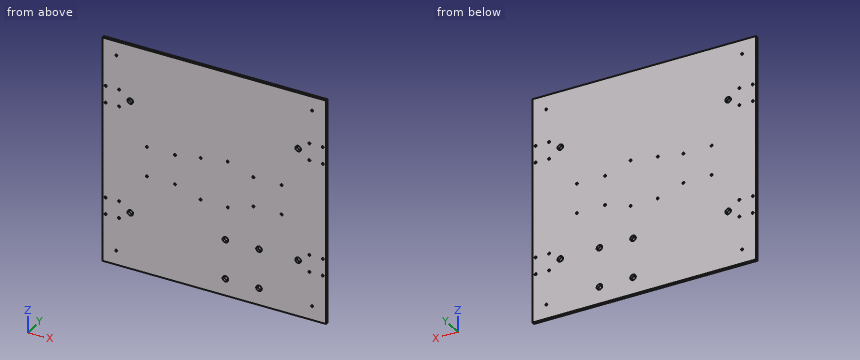
Autodesk Inventor part; units mm, degrees
ref_plane "YZ Plane" through (0, 0, 0) normal (1, 0, 0) x (0, 1, 0)
ref_plane "XZ Plane" through (0, 0, 0) normal (0, 1, 0) x (-1, 0, 0)
ref_plane "XY Plane" through (0, 0, 0) normal (0, 0, 1) x (1, 0, 0)
sketch "草图1" plane through (0, 0, 0) normal (0, 1, 0) x (-1, 0, 0)
  line L0 (200, 200) -> (-200, 200)
  line L1 (-200, 200) -> (-200, -200)
  line L2 (-200, -200) -> (200, -200)
  line L3 (200, -200) -> (200, 200)
  point P0 (0, 0)
  dimension "d0" = 400
  dimension "d1" = 400
extrude "拉伸1" add sketch "草图1" along normal blind 5
sketch "草图2" plane through (0, 5, 0) normal (0, 1, 0) x (1, 0, 0)
  circle A0 centre (175, 175) radius 1.8
  point P0 (0, 0)
  dimension "d4" = 3.6
extrude "拉伸2" cut sketch "草图2" against normal through all
sketch "草图3" plane through (0, 0, 0) normal (0, -1, 0) x (1, 0, 0)
  circle A0 centre (175, 175) radius 1.8
  point P0 (0, 0)
  dimension "d7" = 3.6
extrude "拉伸3" cut sketch "草图3" against normal through all
sketch "草图4" plane through (0, 0, 0) normal (0, -1, 0) x (1, 0, 0)
  circle A0 centre (-175, -175) radius 1.8
  point P0 (0, 0)
  dimension "d10" = 3.6
extrude "拉伸4" cut sketch "草图4" against normal through all
sketch "草图5" plane through (0, 0, 0) normal (0, -1, 0) x (1, 0, 0)
  circle A0 centre (-175, 175) radius 1.8
  point P0 (0, 0)
  dimension "d13" = 3.6
extrude "拉伸5" cut sketch "草图5" against normal through all
sketch "草图6" plane through (0, 0, 0) normal (0, -1, 0) x (1, 0, 0)
  circle A0 centre (-194, -85) radius 1.8
  point P0 (0, 0)
  dimension "d16" = 3.6
extrude "拉伸6" cut sketch "草图6" against normal through all
sketch "草图7" plane through (0, 0, 0) normal (0, -1, 0) x (1, 0, 0)
  circle A0 centre (-170, -85) radius 1.8
  point P0 (0, 0)
  dimension "d19" = 3.6
extrude "拉伸7" cut sketch "草图7" against normal through all
sketch "草图8" plane through (0, 0, 0) normal (0, -1, 0) x (1, 0, 0)
  circle A0 centre (-194, -115) radius 1.8
  point P0 (0, 0)
  dimension "d22" = 3.6
extrude "拉伸8" cut sketch "草图8" against normal through all
sketch "草图9" plane through (0, 0, 0) normal (0, -1, 0) x (1, 0, 0)
  circle A0 centre (-170, -115) radius 1.8
  point P0 (0, 0)
  dimension "d25" = 3.6
extrude "拉伸9" cut sketch "草图9" against normal through all
sketch "草图10" plane through (0, 0, 0) normal (0, -1, 0) x (1, 0, 0)
  circle A0 centre (194, 85) radius 1.8
  point P0 (0, 0)
  dimension "d28" = 3.6
extrude "拉伸10" cut sketch "草图10" against normal through all
sketch "草图11" plane through (0, 0, 0) normal (0, -1, 0) x (1, 0, 0)
  circle A0 centre (194, 115) radius 1.8
  point P0 (0, 0)
  dimension "d31" = 3.6
extrude "拉伸11" cut sketch "草图11" against normal through all
sketch "草图12" plane through (0, 0, 0) normal (0, -1, 0) x (1, 0, 0)
  circle A0 centre (170, 85) radius 1.8
  point P0 (0, 0)
  dimension "d34" = 3.6
extrude "拉伸12" cut sketch "草图12" against normal through all
sketch "草图13" plane through (0, 0, 0) normal (0, -1, 0) x (1, 0, 0)
  circle A0 centre (170, 115) radius 1.8
  point P0 (0, 0)
  dimension "d37" = 3.6
extrude "拉伸13" cut sketch "草图13" against normal through all
sketch "草图14" plane through (0, 0, 0) normal (0, -1, 0) x (1, 0, 0)
  circle A0 centre (194, -85) radius 1.8
  point P0 (0, 0)
  dimension "d40" = 3.6
extrude "拉伸14" cut sketch "草图14" against normal through all
sketch "草图15" plane through (0, 0, 0) normal (0, -1, 0) x (1, 0, 0)
  circle A0 centre (194, -115) radius 1.8
  point P0 (0, 0)
  dimension "d43" = 3.6
extrude "拉伸15" cut sketch "草图15" against normal through all
sketch "草图16" plane through (0, 0, 0) normal (0, -1, 0) x (1, 0, 0)
  circle A0 centre (170, -85) radius 1.8
  point P0 (0, 0)
  dimension "d46" = 3.6
extrude "拉伸16" cut sketch "草图16" against normal through all
sketch "草图17" plane through (0, 0, 0) normal (0, -1, 0) x (1, 0, 0)
  circle A0 centre (170, -115) radius 1.8
  point P0 (0, 0)
  dimension "d49" = 3.6
extrude "拉伸17" cut sketch "草图17" against normal through all
sketch "草图18" plane through (0, 0, 0) normal (0, -1, 0) x (1, 0, 0)
  circle A0 centre (-194, 115) radius 1.8
  point P0 (0, 0)
  dimension "d52" = 3.6
extrude "拉伸18" cut sketch "草图18" against normal through all
sketch "草图19" plane through (0, 0, 0) normal (0, -1, 0) x (1, 0, 0)
  circle A0 centre (-194, 85) radius 1.8
  point P0 (0, 0)
  dimension "d55" = 3.6
extrude "拉伸19" cut sketch "草图19" against normal through all
sketch "草图20" plane through (0, 0, 0) normal (0, -1, 0) x (1, 0, 0)
  circle A0 centre (-170, 115) radius 1.8
  point P0 (0, 0)
  dimension "d58" = 3.6
extrude "拉伸20" cut sketch "草图20" against normal through all
sketch "草图21" plane through (0, 0, 0) normal (0, -1, 0) x (1, 0, 0)
  circle A0 centre (-170, 85) radius 1.8
  point P0 (0, 0)
  dimension "d61" = 3.6
extrude "拉伸21" cut sketch "草图21" against normal through all
sketch "草图22" plane through (0, 0, 0) normal (0, -1, 0) x (1, 0, 0)
  circle A0 centre (150, 100) radius 5
  point P0 (0, 0)
  dimension "d64" = 10
extrude "拉伸22" cut sketch "草图22" against normal through all
sketch "草图23" plane through (0, 0, 0) normal (0, -1, 0) x (1, 0, 0)
  circle A0 centre (150, -100) radius 5
  point P0 (0, 0)
  dimension "d67" = 10
extrude "拉伸23" cut sketch "草图23" against normal through all
sketch "草图24" plane through (0, 0, 0) normal (0, -1, 0) x (1, 0, 0)
  circle A0 centre (-150, 100) radius 5
  point P0 (0, 0)
  dimension "d70" = 10
extrude "拉伸24" cut sketch "草图24" against normal through all
sketch "草图25" plane through (0, 0, 0) normal (0, -1, 0) x (1, 0, 0)
  circle A0 centre (-150, -100) radius 5
  point P0 (0, 0)
  dimension "d73" = 10
extrude "拉伸25" cut sketch "草图25" against normal through all
sketch "草图26" plane through (0, 0, 0) normal (0, -1, 0) x (1, 0, 0)
  circle A0 centre (24.2, 40.9) radius 1.8
  point P0 (0, 0)
  dimension "d76" = 3.6
extrude "拉伸26" cut sketch "草图26" against normal through all
sketch "草图27" plane through (0, 0, 0) normal (0, -1, 0) x (1, 0, 0)
  circle A0 centre (24.2, -40.9) radius 1.8
  point P0 (0, 0)
  dimension "d79" = 3.6
extrude "拉伸27" cut sketch "草图27" against normal through all
sketch "草图28" plane through (0, 0, 0) normal (0, -1, 0) x (1, 0, 0)
  circle A0 centre (-24.2, -40.9) radius 1.8
  point P0 (0, 0)
  dimension "d82" = 3.6
extrude "拉伸28" cut sketch "草图28" against normal through all
sketch "草图29" plane through (0, 0, 0) normal (0, -1, 0) x (1, 0, 0)
  circle A0 centre (-24.2, 33.9) radius 1.8
  point P0 (0, 0)
  dimension "d85" = 3.6
extrude "拉伸29" cut sketch "草图29" against normal through all
sketch "草图32" plane through (0, 0, 0) normal (0, -1, 0) x (1, 0, 0)
  point P0 (0, 0)
sketch "草图34" plane through (0, 0, 0) normal (0, -1, 0) x (1, 0, 0)
  point P0 (0, 0)
sketch "草图35" plane through (0, 0, 0) normal (0, -1, 0) x (1, 0, 0)
  circle A0 centre (-120.4, 26.2) radius 1.8
  point P0 (0, 0)
  dimension "d97" = 3.6
extrude "拉伸33" cut sketch "草图35" against normal through all
sketch "草图36" plane through (0, 0, 0) normal (0, -1, 0) x (1, 0, 0)
  circle A0 centre (-70, 26.2) radius 1.8
  point P0 (0, 0)
  dimension "d100" = 3.6
extrude "拉伸34" cut sketch "草图36" against normal through all
sketch "草图37" plane through (0, 0, 0) normal (0, -1, 0) x (1, 0, 0)
  circle A0 centre (70, 26.2) radius 1.8
  point P0 (0, 0)
  dimension "d103" = 3.6
extrude "拉伸35" cut sketch "草图37" against normal through all
sketch "草图38" plane through (0, 0, 0) normal (0, -1, 0) x (1, 0, 0)
  circle A0 centre (120.4, 26.2) radius 1.8
  point P0 (0, 0)
  dimension "d106" = 3.6
extrude "拉伸36" cut sketch "草图38" against normal through all
sketch "草图39" plane through (0, 0, 0) normal (0, -1, 0) x (1, 0, 0)
  circle A0 centre (-70, -26.2) radius 1.8
  point P0 (0, 0)
  dimension "d109" = 3.6
extrude "拉伸37" cut sketch "草图39" against normal through all
sketch "草图40" plane through (0, 0, 0) normal (0, -1, 0) x (1, 0, 0)
  circle A0 centre (70, -26.2) radius 1.8
  point P0 (0, 0)
  dimension "d112" = 3.6
extrude "拉伸38" cut sketch "草图40" against normal through all
sketch "草图41" plane through (0, 0, 0) normal (0, -1, 0) x (1, 0, 0)
  circle A0 centre (120.4, -26.2) radius 1.8
  point P0 (0, 0)
  dimension "d115" = 3.6
extrude "拉伸39" cut sketch "草图41" against normal through all
sketch "草图42" plane through (0, 0, 0) normal (0, -1, 0) x (1, 0, 0)
  circle A0 centre (-120.4, -26.2) radius 1.8
  point P0 (0, 0)
  dimension "d118" = 3.6
extrude "拉伸40" cut sketch "草图42" against normal through all
sketch "草图43" plane through (0, 0, 0) normal (0, -1, 0) x (1, 0, 0)
  circle A0 centre (20, -100) radius 5
  point P0 (0, 0)
  dimension "d121" = 10
extrude "拉伸41" cut sketch "草图43" against normal through all
sketch "草图44" plane through (0, 0, 0) normal (0, -1, 0) x (1, 0, 0)
  circle A0 centre (80, -100) radius 5
  point P0 (0, 0)
  dimension "d124" = 10
extrude "拉伸42" cut sketch "草图44" against normal through all
sketch "草图45" plane through (0, 0, 0) normal (0, -1, 0) x (1, 0, 0)
  circle A0 centre (20, -170) radius 5
  point P0 (0, 0)
  dimension "d127" = 10
extrude "拉伸43" cut sketch "草图45" against normal through all
sketch "草图46" plane through (0, 0, 0) normal (0, -1, 0) x (1, 0, 0)
  circle A0 centre (80, -170) radius 5
  point P0 (0, 0)
  dimension "d130" = 10
extrude "拉伸44" cut sketch "草图46" against normal through all
sketch "草图47" plane through (0, 0, 0) normal (0, -1, 0) x (1, 0, 0)
  point P0 (0, 0)
equation "\"折弯半径\" = 厚度"
equation "\"折弯释压宽度\" = 厚度"
equation "\"折弯释压深度\" = 0.5 * 厚度"
equation "\"拐角释压尺寸\" = 4 * 厚度"
equation "\"最小余量\" = 2 * 厚度"
equation "\"过渡半径\" = 折弯半径"
equation "\"Jacobi半径尺寸\" = 折弯半径"
equation "\"间隙大小\" = 厚度"
properties part number "下层板"
CAD build for the part. Positions are in the model's coordinates, mm. Coordinates: 2 decimals unless noted, no trailing zeros. Write each loop counter-clockwise with the first axis right and the second up, starting at its lowest first coordinate (ties: lowest second). Pieces come first, ordered by that corner, then holes. Notation, with made-up numbers: (27.5, 62) -> (37.5, 62) arc R9 cw to (37.5, 75) -> close; hole circle Ø6 at (37.5, 70.25). An arc over 180 degrees is marked (long way). Return JSON: item names as keys, results as strings. Group by question number.
Q1. Cut at B-B, the plane x = -150. Give the cut face in (y, z).
Q2. Drill centre lines: line 1 (X direction, y = 1.35, z = 115); line 2 (Z direction, x = 120.4, y = 2.8); line 3 (Z direction, x = -170, y = 4.35). Where is each one in solid material? Low to high.
Q3. Cut at A-A, the plane z = 100. Give the cut face in (x, y).
Returned:
{
 "1": {"outline": "(0, -200) -> (5, -200) -> (5, -105) -> (0, -105) -> close; (0, -95) -> (5, -95) -> (5, 95) -> (0, 95) -> close; (0, 105) -> (5, 105) -> (5, 200) -> (0, 200) -> close"},
 "2": {"line 1": "x = -200 to -195.8, -192.2 to -171.8, -168.2 to 168.2, 171.8 to 192.2, 195.8 to 200", "line 2": "z = -200 to -28, -24.4 to 24.4, 28 to 200", "line 3": "z = -200 to -116.8, -113.2 to -86.8, -83.2 to 83.2, 86.8 to 113.2, 116.8 to 200"},
 "3": {"outline": "(-200, 0) -> (-155, 0) -> (-155, 5) -> (-200, 5) -> close; (-145, 0) -> (145, 0) -> (145, 5) -> (-145, 5) -> close; (155, 0) -> (200, 0) -> (200, 5) -> (155, 5) -> close"}
}
